Geometry: final body of the model. Coordinates: model frame, mm. A direction names the side the tool comes from. Round coordinates to 2 decimals unless told otherwise and drop trailing zeros. Loops run counter-clockwise (first coordinate to the right, second up) from the corner with the lowest first, then second, coordinate; pieces in that order, holes last. Notation, with made-up numbers: M -15.75,82 L 18.25,82 A13 cw 18.25,93 Z; hole C -13,-27.5 d8. An arc over 180 degrees is marked long. Return JSON: item names as keys, results as strings.
from build123d import *

# Parameters (mm, degrees)
SALIENTE_EXTRUIR1_DEPTH   = 3
SALIENTE_EXTRUIR1_2_DEPTH = 3
SALIENTE_EXTRUIR2_DEPTH   = 6
SALIENTE_EXTRUIR2_2_DEPTH = 6
SALIENTE_EXTRUIR3_DEPTH   = 3.5
SALIENTE_EXTRUIR3_2_DEPTH = 3.5
SALIENTE_EXTRUIR4_DEPTH   = 3
SALIENTE_EXTRUIR5_DEPTH   = 3
CROQUIS3_R                = 1.575
CORTAR_EXTRUIR1_DEPTH     = 2.5
CROQUIS4_W                = 3.383823373
CROQUIS4_H                = 8.6242578
CROQUIS4_W_2              = 3.249859327
CROQUIS4_H_2              = 9.348028676
CROQUIS4_W_3              = 4.000427531
CROQUIS4_H_3              = 6.045673659
CROQUIS4_W_4              = 2.224540958
SALIENTE_EXTRUIR6_DEPTH   = 1


with BuildPart() as part:
    # Croquis1 → Saliente-Extruir1 (new body)
    with BuildSketch(Plane(origin=(0, 0, 0), x_dir=(1, 0, 0), z_dir=(0, 1, 0))):
        Polygon((-10, -2.25), (-10, -3.75), (10, -3.75), (10, -3.630117405), (9.771655233, -3.535533906), (9.239169654, -2.25), align=None)
    extrude(amount=SALIENTE_EXTRUIR1_DEPTH)



with BuildPart() as body_2:
    # Croquis1 → Saliente-Extruir1 2 (new body)
    with BuildSketch(Plane(origin=(0, 0, 0), x_dir=(1, 0, 0), z_dir=(0, 1, 0))):
        Polygon((-10, 3.75), (-10, 2.25), (9.239169654, 2.25), (9.771655233, 3.535533906), (10, 3.630117405), (10, 3.75), align=None)
    extrude(amount=SALIENTE_EXTRUIR1_2_DEPTH)


with BuildPart() as body_3:
    # Croquis1_3 → Saliente-Extruir2 (new body)
    with BuildSketch(Plane(origin=(0, 0, 0), x_dir=(1, 0, 0), z_dir=(0, 1, 0))):
        Polygon((9.771655233, 3.535533906), (10.478762014, 2.828427125), (13.307189139, 4), (13.307189139, 5), align=None)
    extrude(amount=SALIENTE_EXTRUIR2_DEPTH)


with BuildPart() as body_4:
    # Croquis1_3 → Saliente-Extruir2 2 (new body)
    with BuildSketch(Plane(origin=(0, 0, 0), x_dir=(1, 0, 0), z_dir=(0, 1, 0))):
        Polygon((16.842723045, -3.535533906), (18.307189139, 0), (17.307189139, 0), (16.135616264, -2.828427125), align=None)
    extrude(amount=SALIENTE_EXTRUIR2_2_DEPTH)


with BuildPart() as body_5:
    # Croquis1_4 → Saliente-Extruir3 (new body)
    with BuildSketch(Plane(origin=(0, 0, 0), x_dir=(1, 0, 0), z_dir=(0, 1, 0))):
        Polygon((16.842723045, 3.535533906), (16.135616264, 2.828427125), (13.307189139, 4), (13.307189139, 5), align=None)
    extrude(amount=SALIENTE_EXTRUIR3_DEPTH)


with BuildPart() as body_6:
    # Croquis1_4 → Saliente-Extruir3 2 (new body)
    with BuildSketch(Plane(origin=(0, 0, 0), x_dir=(1, 0, 0), z_dir=(0, 1, 0))):
        Polygon((13.307189139, -5), (13.307189139, -4), (16.135616264, -2.828427125), (16.842723045, -3.535533906), align=None)
    extrude(amount=SALIENTE_EXTRUIR3_2_DEPTH)


with BuildPart() as body_7:
    # Croquis1_5 → Saliente-Extruir4 (new body)
    with BuildSketch(Plane(origin=(0, 0, 0), x_dir=(1, 0, 0), z_dir=(0, 1, 0))):
        Polygon((10, -3.307189139), (10, -3.630117405), (13.307189139, -5), (13.307189139, -4), (10.478762014, -2.828427125), align=None)
        Polygon((18.307189139, 0), (17.307189139, 0), (16.135616264, 2.828427125), (16.842723045, 3.535533906), align=None)
        Polygon((9.771655233, -3.535533906), (10, -3.630117405), (10, -3.307189139), align=None)
    extrude(amount=SALIENTE_EXTRUIR4_DEPTH)


with BuildPart() as part_1:
    add(part.part)

    add(body_2.part)  # Saliente-Extruir5 merges body 2

    add(body_3.part)  # Saliente-Extruir5 merges body 3

    add(body_4.part)  # Saliente-Extruir5 merges body 4

    add(body_5.part)  # Saliente-Extruir5 merges body 5

    add(body_6.part)  # Saliente-Extruir5 merges body 6

    add(body_7.part)  # Saliente-Extruir5 merges body 7
    # Croquis2 → Saliente-Extruir5 (add)
    with BuildSketch(Plane.XZ):
        Polygon((9.239169654, 2.25), (-10, 2.25), (-10, -3.75), (10, -3.75), (10, -3.630117405), (9.771655233, -3.535533906), (8.307189139, 0), align=None)
        Polygon((13.307189139, 5), (10, 3.630117405), (10, -3.630117405), (13.307189139, -5), (16.842723045, -3.535533906), (18.307189139, 0), (16.842723045, 3.535533906), align=None)
        Polygon((10, -3.630117405), (10, 3.630117405), (9.771655233, 3.535533906), (9.239169654, 2.25), (8.307189139, 0), (9.771655233, -3.535533906), align=None)
        Polygon((9.239169654, 2.25), (9.771655233, 3.535533906), (10, 3.630117405), (10, 3.75), (-10, 3.75), (-10, 2.25), align=None)
    extrude(amount=SALIENTE_EXTRUIR5_DEPTH)

    # Croquis3 → Cortar-Extruir1 (cut)
    with BuildSketch(Plane.XZ.offset(3)):
        with Locations(Location((4.333266607, 0, 0), (0, 0, 270))):
            Circle(CROQUIS3_R)
    extrude(amount=-CORTAR_EXTRUIR1_DEPTH, mode=Mode.SUBTRACT)

    # Croquis4 → Saliente-Extruir6 (add)
    with BuildSketch(Plane(origin=(0, 3, 0), x_dir=(1, 0, 0), z_dir=(0, 1, 0))):
        with Locations((8.211188083, -0.151851299)):
            Rectangle(CROQUIS4_W, CROQUIS4_H)
        with Locations((4.390228963, -0.260399993)):
            Rectangle(CROQUIS4_W_2, CROQUIS4_H_2)
        with Locations((0.297050365, -0.094855663)):
            Rectangle(CROQUIS4_W_3, CROQUIS4_H_3)
        with Locations((-5.85391415, -0.094855663)):
            Rectangle(CROQUIS4_W_4, CROQUIS4_H_3)
    extrude(amount=SALIENTE_EXTRUIR6_DEPTH)


solid = part_1.part
Q1. Section query A-A (y = 5.5). Output: boundary loops of the cut face in (x, z).
Determined:
{"outline": "M 9.77,-3.54 L 13.31,-5 L 13.31,-4 L 10.48,-2.83 Z; M 16.14,2.83 L 17.31,0 L 18.31,0 L 16.84,3.54 Z"}
Q2. Reachability of faces 4 (the flat face through (14.702, 1.726, 3.422)), 5 (the flat face through (-4.742, 3.5, 0.1)), 6 (the flat face through (0.3, 3.5, -2.928)) from +Z, -Z, +X, -X, +Y, -Y: full face, straight path, thin tool, end or side. Return the list, or none.
Determined:
{"face 4": "+Y", "face 5": "+Z, -Z, +Y", "face 6": "-Z, -X, +Y"}
Q3. Pull-direction query (Y, two-part tool) for faces 1 (the flat face through (8, 4, 0)), 2 (the flat face through (8, 3, 0)), 3 (the flat face through (11.873, 2.958, -3.406)); classes: pulls with the +Y half, pulls with the -Y half, needs draft (parallel to the pull), parting line crosses it, or undercut.
Determined:
{"face 1": "pulls with the +Y half", "face 2": "undercut", "face 3": "needs draft"}
Q4. Pin query (flat end, axial travel): pin 1 (1.6 mm diameter, centred on x = 4.5, z = 0.5, fed in from -Y); pin 2 (1.1 mm diameter, centred on y = 3.5, z = -1, fed in from -X); pin 3 (1.1 mm diameter, centred on x = 0.5, y = 3.5, fed in from +Z). Return the tip coordinate at first contact, or that it passes through.
Determined:
{"pin 1": "stops at y = -0.5", "pin 2": "stops at x = -6.97", "pin 3": "stops at z = 3.75"}
Q5. Section query D-D (z = -0.5). Output: boundary loops of the cut face in (x, y), plus the area to 3 significant figures.
Determined:
{"outline": "M -10,-3 L 2.84,-3 L 2.84,-0.5 L 5.83,-0.5 L 5.83,-3 L 18.1,-3 L 18.1,3 L 17.1,3 L 17.1,0 L -10,0 Z; M -6.97,3 L -4.74,3 L -4.74,4 L -6.97,4 Z; M -1.7,3 L 2.3,3 L 2.3,4 L -1.7,4 Z; M 2.77,3 L 6.02,3 L 6.02,4 L 2.77,4 Z; M 6.52,3 L 9.9,3 L 9.9,4 L 6.52,4 Z", "area": "92.7 mm^2"}
Q6. Section query B-B (x = -2). Output: boundary loops of the cut face in (y, z).
Determined:
{"outline": "M -3,-3.75 L 3,-3.75 L 3,-2.25 L 0,-2.25 L 0,2.25 L 3,2.25 L 3,3.75 L -3,3.75 Z"}
Q7. Section query C-C (x = 8.5). Output: boundary loops of the cut face in (y, z), plus the area to 3 significant figures.
Determined:
{"outline": "M -3,-3.75 L 3,-3.75 L 3,-4.16 L 4,-4.16 L 4,4.46 L 3,4.46 L 3,3.75 L -3,3.75 Z; hole M 0,-2.25 L 3,-2.25 L 3,2.25 L 0,2.25 Z", "area": "40.1 mm^2"}
Q8. Material intervals for L1, parallel to Z at x = -4.75, y = 0.75; L2, parallel to X at y = -1.5, z = 0; L3, parallel to Y at x = 3.25, z = 2, sorted ascending.
Determined:
{"L1": "z = -3.75 to -2.25, 2.25 to 3.75", "L2": "x = -10 to 2.76, 5.91 to 18.31", "L3": "y = -3 to 0, 3 to 4"}
